Autodesk Inventor part; units mm, degrees
ref_plane "YZ Plane" through (0, 0, 0) normal (1, 0, 0) x (0, 1, 0)
ref_plane "XZ Plane" through (0, 0, 0) normal (0, 1, 0) x (-1, 0, 0)
ref_plane "XY Plane" through (0, 0, 0) normal (0, 0, 1) x (1, 0, 0)
sketch "Sketch1" plane through (0, 0, 0) normal (0, 0, 1) x (1, 0, 0)
  line L0 (-12.7, -25.4) -> (12.7, -25.4)
  line L1 (12.7, -25.4) -> (12.7, 25.4)
  line L2 (12.7, 25.4) -> (-12.7, 25.4)
  line L3 (-12.7, 25.4) -> (-12.7, -25.4)
  line L4 (-12.7, -25.4) -> (12.7, 25.4) construction
  line L5 (12.7, -25.4) -> (-12.7, 25.4) construction
  line L6 (-11.1125, -23.8125) -> (11.1125, -23.8125)
  line L7 (11.1125, -23.8125) -> (11.1125, 23.8125)
  line L8 (11.1125, 23.8125) -> (-11.1125, 23.8125)
  line L9 (-11.1125, 23.8125) -> (-11.1125, -23.8125)
  point P0 (0, 0)
  dimension "d0" = 25.4
  dimension "d1" = 50.8
  dimension "d2" = 1.5875
extrude "BaseTube" add sketch "Sketch1" along normal mid plane 228.6
sketch "TopPoint" plane through (-12.7, 25.4, 114.3) normal (0, 1, 0) x (1, 0, 0)
  line L0 (25.4, 0) -> (0, 0)
  line L1 (0, 228.6) -> (0, 0)
  point P0 (12.7, 12.7)
  dimension "TLE_" = 12.7
  dimension "TWE_" = 12.7
sketch "SidePoint" plane through (12.7, -25.4, 114.3) normal (1, 0, 0) x (0, 0, -1)
  line L0 (0, 0) -> (0, 50.8)
  line L1 (228.6, 50.8) -> (0, 50.8)
  point P0 (88.9, 44.45)
  dimension "SLE_" = 88.9
  dimension "SWE_" = 6.35
hole "TopHole" at (0, 25.4, 101.6) direction (0, -1, 0) diameter 4.9784 end through all
hole "SideHole" [suppressed]
pattern_linear "TopPattern" count 9 spacing 12.7 along (0, 0, -1) of "TopHole"
pattern_linear "SidePattern" [suppressed]
mirror "TopMirror" about plane through (0, 0, 0) normal (0, 0, 1) of "TopHole", "TopPattern"
mirror "SideMirror" [suppressed]
sketch "Sketch4" plane through (-12.7, 25.4, 114.3) normal (0, 1, 0) x (1, 0, 0)
  line L0 (25.4, 228.6) -> (25.4, 0)
  line L1 (25.4, 0) -> (0, 0)
  line L2 (0, 228.6) -> (25.4, 228.6)
  line L3 (0, 228.6) -> (0, 0)
  line L4 (0, 0) -> (25.4, 25.4)
  line L5 (0, 228.6) -> (25.4, 203.2)
  dimension "d36" = 25.4
extrude "CornerCut" [suppressed]
sketch "Sketch5" plane through (12.7, -25.4, 114.3) normal (1, 0, 0) x (0, 0, -1)
  circle A0 centre (31.75, 25.4) radius 14.2875
  line L0 (0, 0) -> (0, 50.8)
  point P0 (0, 25.4)
  dimension "d39" = 28.575
  dimension "d40" = 31.75
extrude "FrontBearingHole" [suppressed]
sketch "Sketch6" plane through (12.7, -25.4, 114.3) normal (1, 0, 0) x (0, 0, -1)
  circle A0 centre (196.85, 25.4) radius 14.2875
  line L0 (228.6, 50.8) -> (228.6, 0)
  point P0 (228.6, 25.4)
  dimension "d43" = 28.575
  dimension "d44" = 31.75
extrude "BackBearingHole" [suppressed]
sketch "6wd" plane through (12.7, -25.4, 114.3) normal (1, 0, 0) x (0, 0, -1)
  circle A0 centre (-66.668, 25.4) radius 14.2875
  circle A1 centre (114.3, 23.8125) radius 14.2875
  circle A2 centre (295.268, 25.4) radius 14.2875
  line L0 (228.6, 50.8) -> (0, 50.8)
  line L1 (228.6, 0) -> (0, 0) construction
  arc A3 (-66.5085, 43.5907) -> (-66.8276, 7.2093) centre (-66.668, 25.4) ccw construction
  arc A4 (114.1404, 5.6218) -> (114.4596, 42.0032) centre (114.3, 23.8125) ccw construction
  line L2 (-66.5085, 43.5907) -> (114.4596, 42.0032) construction
  line L3 (114.1404, 5.6218) -> (-66.8276, 7.2093) construction
  circle A5 centre (-66.668, 25.4) radius 50.8 construction
  circle A6 centre (114.3, 23.8125) radius 50.8 construction
  circle A7 centre (295.268, 25.4) radius 50.8 construction
  point P0 (-49.8301, 8.562)
  point P1 (97.462, 40.6505)
  point P2 (278.4301, 42.238)
  point P3 (-42.8555, 25.4)
  point P4 (-49.8301, 42.238)
  point P5 (-66.668, 49.2125)
  point P6 (-83.506, 42.238)
  point P7 (-90.4805, 25.4)
  point P8 (-83.506, 8.562)
  point P9 (-66.668, 1.5875)
  point P10 (90.4875, 23.8125)
  point P11 (97.462, 6.9745)
  point P12 (114.3, 0)
  point P13 (131.138, 6.9745)
  point P14 (138.1125, 23.8125)
  point P15 (131.138, 40.6505)
  point P16 (114.3, 47.625)
  point P17 (271.4555, 25.4)
  point P18 (278.4301, 8.562)
  point P19 (295.268, 1.5875)
  point P20 (312.106, 8.562)
  point P21 (319.0805, 25.4)
  point P22 (312.106, 42.238)
  point P23 (295.268, 49.2125)
  point P24 (114.3, 50.8)
  point P25 (-123.818, 25.4)
  point P26 (57.15, 23.8125)
  point P27 (238.118, 25.4)
  point P28 (-9.518, 25.4)
  point P29 (171.45, 23.8125)
  point P30 (352.418, 25.4)
  point P31 (-28.568, 26.9875)
  point P32 (257.168, 26.9875)
  point P33 (152.4, 26.9875)
  point P34 (76.2, 26.9875)
  dimension "d47" = 28.575
  dimension "d50" = 315
  dimension "d52" = 25.4
  dimension "d55" = 315
  dimension "d59" = 315
  dimension "d61" = 23.8125
  dimension "d62" = 23.8125
  dimension "d63" = 23.8125
  dimension "d64" = 26.9875
  dimension "d68" = 36.3828
  dimension "d69" = 57.15
  dimension "d70" = 180.975
  dimension "d71" = 57.15
  dimension "d72" = 180.975
  dimension "d73" = 180.975
  dimension "d74" = 101.6
  dimension "d131" = 180
  dimension "d133" = 114.3
  dimension "d136" = 360
  dimension "d140" = 360
  dimension "d142" = 114.3
  dimension "d143" = 114.3
  dimension "d186" = 38.1
  dimension "d187" = 38.1
  dimension "d188" = 38.1
  dimension "d189" = 38.1
  dimension "d190" = 23.8125
extrude "6wdBearings" [suppressed]
hole "6wdBearingBlocks" [suppressed]
sketch "8wd" plane through (12.7, -25.4, 114.3) normal (1, 0, 0) x (0, 0, -1)
  circle A0 centre (-71.3968, 26.9875) radius 14.2875
  circle A1 centre (52.3875, 23.8125) radius 14.2875
  circle A2 centre (176.2125, 23.8125) radius 14.2875
  circle A3 centre (299.9968, 26.9875) radius 14.2875
  line L0 (228.6, 50.8) -> (0, 50.8)
  arc A4 (-70.9303, 45.1729) -> (-71.8632, 8.8021) centre (-71.3968, 26.9875) ccw construction
  arc A5 (51.9211, 5.6271) -> (52.8539, 41.9979) centre (52.3875, 23.8125) ccw construction
  line L1 (-70.9303, 45.1729) -> (52.8539, 41.9979) construction
  line L2 (51.9211, 5.6271) -> (-71.8632, 8.8021) construction
  arc A6 (176.2125, 5.6211) -> (176.2125, 42.0039) centre (176.2125, 23.8125) ccw construction
  arc A7 (52.3875, 42.0039) -> (52.3875, 5.6211) centre (52.3875, 23.8125) ccw construction
  line L3 (52.3875, 42.0039) -> (176.2125, 42.0039) construction
  line L4 (52.3875, 5.6211) -> (176.2125, 5.6211) construction
  line L5 (114.3, 50.8) -> (114.3, 0) construction
  line L6 (0, 0) -> (228.6, 0)
  circle A8 centre (-71.3968, 26.9875) radius 50.8 construction
  circle A9 centre (52.3875, 23.8125) radius 50.8 construction
  circle A10 centre (176.2125, 23.8125) radius 50.8 construction
  circle A11 centre (299.9968, 26.9875) radius 50.8 construction
  line L7 (0, 0) -> (0, 50.8)
  line L8 (228.6, 50.8) -> (228.6, 0)
  point P0 (-71.3968, 50.8)
  point P1 (52.3875, 47.625)
  point P2 (176.2125, 47.625)
  point P3 (299.9968, 50.8)
  point P4 (-88.2348, 43.8255)
  point P5 (-95.2093, 26.9875)
  point P6 (-88.2348, 10.1495)
  point P7 (-71.3968, 3.175)
  point P8 (-54.5588, 10.1495)
  point P9 (-47.5843, 26.9875)
  point P10 (-54.5588, 43.8255)
  point P11 (35.5495, 40.6505)
  point P12 (28.575, 23.8125)
  point P13 (35.5495, 6.9745)
  point P14 (52.3875, 0)
  point P15 (69.2255, 6.9745)
  point P16 (76.2, 23.8125)
  point P17 (69.2255, 40.6505)
  point P18 (159.3745, 40.6505)
  point P19 (152.4, 23.8125)
  point P20 (159.3745, 6.9745)
  point P21 (176.2125, 0)
  point P22 (193.0505, 6.9745)
  point P23 (200.025, 23.8125)
  point P24 (193.0505, 40.6505)
  point P25 (283.1588, 43.8255)
  point P26 (276.1843, 26.9875)
  point P27 (283.1588, 10.1495)
  point P28 (299.9968, 3.175)
  point P29 (316.8348, 10.1495)
  point P30 (323.8093, 26.9875)
  point P31 (316.8348, 43.8255)
  point P32 (-128.5468, 26.9875)
  point P33 (-14.2468, 26.9875)
  point P34 (-4.7625, 23.8125)
  point P35 (119.0625, 23.8125)
  point P36 (242.8468, 26.9875)
  point P37 (109.5375, 23.8125)
  point P38 (233.3625, 23.8125)
  point P39 (357.1468, 26.9875)
  point P40 (-33.3299, 25.4)
  point P41 (14.2875, 25.4)
  point P42 (90.4875, 25.4)
  point P43 (138.1125, 25.4)
  point P44 (214.3125, 25.4)
  point P45 (261.9299, 25.4)
  dimension "d84" = 28.575
  dimension "d86" = 26.9875
  dimension "d87" = 23.8125
  dimension "d88" = 23.8125
  dimension "d89" = 23.8125
  dimension "d90" = 23.8125
  dimension "d93" = 360
  dimension "d97" = 360
  dimension "d101" = 360
  dimension "d105" = 360
  dimension "d107" = 36.3828
  dimension "d108" = 57.15
  dimension "d109" = 123.825
  dimension "d110" = 57.15
  dimension "d111" = 123.825
  dimension "d112" = 123.825
  dimension "d113" = 36.3828
  dimension "d114" = 57.15
  dimension "d115" = 123.825
  dimension "d116" = 57.15
  dimension "d117" = 123.825
  dimension "d118" = 61.9125
  dimension "d119" = 101.6
  dimension "d206" = 23.8125
  dimension "d211" = 360
  dimension "d213" = 114.3
  dimension "d216" = 360
  dimension "d218" = 114.3
  dimension "d221" = 360
  dimension "d223" = 114.3
  dimension "d226" = 360
  dimension "d228" = 114.3
  dimension "d285" = 25.4
  dimension "d286" = 38.1
  dimension "d287" = 38.1
  dimension "d288" = 38.1
  dimension "d289" = 38.1
  dimension "d290" = 38.1
  dimension "d291" = 38.1
extrude "8wdBearings" [suppressed]
hole "8wdBearingBlocks" [suppressed]
sketch "6wdPoints" plane through (-12.7, -25.4, 114.3) normal (-1, 0, 0) x (0, 0, 1)
  point P0 (123.818, 25.4)
  point P1 (9.518, 25.4)
  point P2 (-57.15, 23.8125)
  point P3 (-171.45, 23.8125)
  point P4 (-238.118, 25.4)
  point P5 (-352.418, 25.4)
  point P6 (28.568, 26.9875)
  point P7 (-76.2, 26.9875)
  point P8 (-152.4, 26.9875)
  point P9 (-257.168, 26.9875)
hole "FL6wdGB" [suppressed]
hole "ML6wdGB" [suppressed]
hole "BL6wdGB" [suppressed]
hole "FR6wdGB" [suppressed]
hole "MR6wdGB" [suppressed]
hole "BR6wdGB" [suppressed]
hole "CL6wd" [suppressed]
hole "CR6wd" [suppressed]
sketch "Sketch10" plane through (-12.7, -25.4, 114.3) normal (-1, 0, 0) x (0, 0, 1)
  point P0 (128.5468, 26.9875)
  point P1 (14.2468, 26.9875)
  point P2 (4.7625, 23.8125)
  point P3 (-109.5375, 23.8125)
  point P4 (-119.0625, 23.8125)
  point P5 (-233.3625, 23.8125)
  point P6 (-242.8468, 26.9875)
  point P7 (-357.1468, 26.9875)
hole "FL8wdGB" [suppressed]
hole "FMdL8wdGB" [suppressed]
hole "BMdL8wdGB" [suppressed]
hole "BL8wdGB" [suppressed]
hole "FR8wdGB" [suppressed]
hole "FMdR8wdGB" [suppressed]
hole "BMdR8wdGB" [suppressed]
hole "BR8wdGB" [suppressed]
hole "CL8wd" [suppressed]
sketch "Sketch11" plane through (-12.7, -25.4, 114.3) normal (-1, 0, 0) x (0, 0, 1)
  line L0 (-228.6, 50.8) -> (0, 50.8)
  line L1 (0, 0) -> (0, 50.8)
  line L2 (0, 0) -> (-228.6, 0)
  line L3 (-228.6, 50.8) -> (-228.6, 0)
  point P0 (33.3299, 25.4)
  point P1 (-14.2875, 25.4)
  point P2 (-90.4875, 25.4)
  point P3 (-138.1125, 25.4)
  point P4 (-214.3125, 25.4)
  point P5 (-261.9299, 25.4)
hole "CR8wd" [suppressed]
sketch "Sketch12" plane through (-12.7, -25.4, 114.3) normal (-1, 0, 0) x (0, 0, 1)
  circle A0 centre (-152.4, 44.45) radius 2.4892
  circle A1 centre (-152.4, 31.75) radius 2.4892
  circle A2 centre (-152.4, 19.05) radius 2.4892
  circle A3 centre (-152.4, 6.35) radius 2.4892
  circle A4 centre (-88.9, 44.45) radius 2.4892
  circle A5 centre (-88.9, 31.75) radius 2.4892
  circle A6 centre (-88.9, 19.05) radius 2.4892
  circle A7 centre (-88.9, 6.35) radius 2.4892
  point P0 (-88.9, 31.75)
hole "Hole23" [suppressed]
equation "\"d0\" = Width"
equation "\"d1\" = Height"
equation "\"d2\" = Wall"
equation "\"d3\" = Length"
equation "\"d6\" = HoleSize"
equation "\"d73\" = d72"
equation "\"d77\" = HoleSize"
equation "\"Height\" = 50.8"
equation "\"Width\" = 25.4"
equation "\"Wall\" = 1.5875"
equation "\"Length\" = 228.6"
equation "\"Top_Lengthwise_Space\" = 12.7"
equation "\"Top_Widthwise_Space\" = 12.7"
equation "\"Top_Lengthwise_Edge\" = 12.7"
equation "\"Top_Widthwise_Edge\" = 12.7"
equation "\"Side_Lengthwise_Edge\" = 88.9"
equation "\"Side_Widthwise_Edge\" = 12.7"
equation "\"Side_Lengthwise_Space\" = 12.7"
equation "\"Side_Widthwise_Space\" = 12.7"
properties part number "GreyT Claw 2 Main Tube 9 Gusset" material "Aluminum 6061"
CAD build for the part. Positions are in the model's coordinates, mm. Coordinates: 2 decimals unless noted, no trailing zeros. Order: outer loops, then holes, each group sorted by start corner. A loop starts at its lowest first (then second) coordinate and runs counter-clockwise, first axis right, second up.
Item 1: Drill centre lines: L1, parallel to Y at x = -6.5, z = -78.5; L2, parallel to X at y = -24.3, z = 25.4; L3, parallel to X at y = 14, z = -25.5. Where is each one in solid material? Low to high.
Check sheet entries:
L1: y = -25.4 to -23.81, 23.81 to 25.4
L2: x = -12.7 to -2.49, 2.49 to 12.7
L3: x = -12.7 to -11.11, 11.11 to 12.7
Item 2: Pin check, flat tip, straight feed: pin 1 Ø12 at (x, y) = (-5, 19.5) entering from +Z. Stop position of the tip, or through.
Check sheet entries:
pin 1: stops at z = 114.3
Item 3: Band-saw the part on C-C on y = 16.5. List the corners of the cut face in (x, z), plus the area to 3 significant figures.
Check sheet entries:
outline: (-12.7, -114.3) - (-11.11, -114.3) - (-11.11, 114.3) - (-12.7, 114.3) - close; (11.11, -114.3) - (12.7, -114.3) - (12.7, 114.3) - (11.11, 114.3) - close
area: 726 mm2
Item 4: Band-saw the part on D-D on z = -50.5. List the corners of the cut face in (x, y), plus the area to 3 significant figures.
Check sheet entries:
outline: (-12.7, -25.4) - (-2.47, -25.4) - (-2.47, -23.81) - (-11.11, -23.81) - (-11.11, 23.81) - (-2.47, 23.81) - (-2.47, 25.4) - (-12.7, 25.4) - close; (2.47, -25.4) - (12.7, -25.4) - (12.7, 25.4) - (2.47, 25.4) - (2.47, 23.81) - (11.11, 23.81) - (11.11, -23.81) - (2.47, -23.81) - close
area: 216 mm2
Item 5: Band-saw the part on B-B on z = -12.7. List the corners of the cut face in (x, y), plus the area to 3 significant figures.
Check sheet entries:
outline: (-12.7, -25.4) - (-2.49, -25.4) - (-2.49, -23.81) - (-11.11, -23.81) - (-11.11, 23.81) - (-2.49, 23.81) - (-2.49, 25.4) - (-12.7, 25.4) - close; (2.49, -25.4) - (12.7, -25.4) - (12.7, 25.4) - (2.49, 25.4) - (2.49, 23.81) - (11.11, 23.81) - (11.11, -23.81) - (2.49, -23.81) - close
area: 216 mm2
Item 6: Two-plate mould, pull along Y, no slides. Class faces 1 (the face through (11.112, 0, -2)), 2 (the face through (3, 23.812, -2)), 3 (the face through (-3, 25.4, -2)), 4 (the face through (-11.3, 2, 114.3)): +Y half, -Y half, draft (parallel to the pull), parting line (faces both ways), or undercut.
Check sheet entries:
face 1: undercut
face 2: undercut
face 3: +Y half
face 4: draft
Item 7: Band-saw the part on A-A on x = -6.75. List the corners of the cut face in (y, z), plus the area to 3 significant figures.
Check sheet entries:
outline: (-25.4, -114.3) - (-23.81, -114.3) - (-23.81, 114.3) - (-25.4, 114.3) - close; (23.81, -114.3) - (25.4, -114.3) - (25.4, 114.3) - (23.81, 114.3) - close
area: 726 mm2
